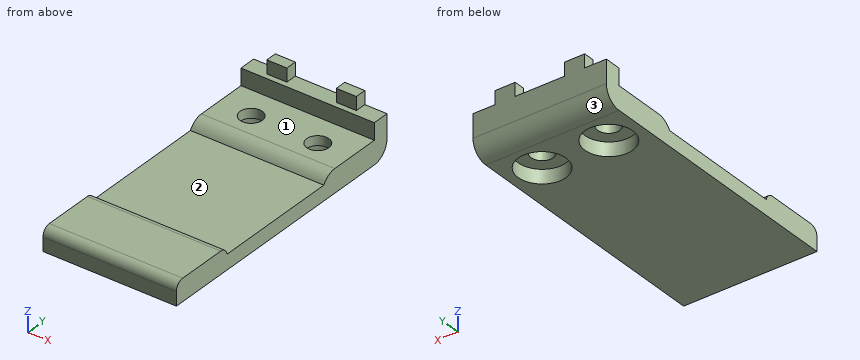
from build123d import *

# Parameters (mm, degrees)
F0_W        = 24
F0_H        = 12
F0_H_2      = 23
F0_R        = 4.3
F0_H_3      = 3
F1_DEPTH    = 2.7
F0_R_2      = 2
F2_DEPTH    = 4.2
F3_DEPTH    = 2.5
F4_DEPTH    = 7.2
F5_W        = 3.6
F5_H        = 2
F6_DEPTH    = 2.4
F7_T1_DEPTH = 39
F7_T3_DEPTH = 36.9903810568
F8_DEPTH    = 4
F9_T1_DEPTH = 31.4330343737
F9_T3_DEPTH = 31.5


# Not quite as in the source:
# - a fillet or chamfer that OpenCascade refuses, or shapes differently, is made with other operations: its cross-section is extruded or revolved along the edge and cut away or added


with BuildPart() as f1:
    # F0 (on Top) → F1 (new body)
    with BuildSketch(Plane.XY):
        with Locations((12, -44)):
            Rectangle(F0_W, F0_H)
        with Locations((12, -26.5)):
            Rectangle(F0_W, F0_H_2)
        with Locations((12, -9)):
            Rectangle(F0_W, F0_H)
        with Locations((6, -8.5)):
            Circle(F0_R, mode=Mode.SUBTRACT)
        with Locations((18, -8.5)):
            Circle(F0_R, mode=Mode.SUBTRACT)
        with Locations((12, -1.5)):
            Rectangle(F0_W, F0_H_3)
    extrude(amount=F1_DEPTH)

    # F0 (on Top) → F2 (join)
    with BuildSketch(Plane.XY):
        with Locations((12, -1.5)):
            Rectangle(F0_W, F0_H_3)
        with Locations((12, -9)):
            Rectangle(F0_W, F0_H)
        with Locations((6, -8.5)):
            Circle(F0_R, mode=Mode.SUBTRACT)
        with Locations((18, -8.5)):
            Circle(F0_R, mode=Mode.SUBTRACT)
        with Locations((6, -8.5)):
            Circle(F0_R)
        with Locations((6, -8.5)):
            Circle(F0_R_2, mode=Mode.SUBTRACT)
        with Locations((18, -8.5)):
            Circle(F0_R)
        with Locations((18, -8.5)):
            Circle(F0_R_2, mode=Mode.SUBTRACT)
    extrude(amount=F2_DEPTH)

    # F0 (on Top) → F3 (cut)
    with BuildSketch(Plane.XY):
        with Locations((6, -8.5)):
            Circle(F0_R)
        with Locations((6, -8.5)):
            Circle(F0_R_2, mode=Mode.SUBTRACT)
        with Locations((18, -8.5)):
            Circle(F0_R)
        with Locations((18, -8.5)):
            Circle(F0_R_2, mode=Mode.SUBTRACT)
    extrude(amount=F3_DEPTH, mode=Mode.SUBTRACT)

    # F0 (on Top) → F4 (join)
    with BuildSketch(Plane.XY):
        with Locations((12, -1.5)):
            Rectangle(F0_W, F0_H_3)
    extrude(amount=F4_DEPTH)

    # F5 (on face) → F6 (join)
    with BuildSketch(Plane.XY.offset(7.2)):
        with Locations((5.7, -1)):
            Rectangle(F5_W, F5_H)
        with Locations((18.2, -1)):
            Rectangle(F5_W, F5_H)
    extrude(amount=F6_DEPTH)

    # F7: fillet of radius 3 on 2 edges, made by hand

    # F7_s2 → F7_t1 (cut)
    with BuildSketch(Plane.YZ.offset(-7.5)):
        with BuildLine():
            ThreePointArc((-3, 0), (-0.8786796564, 0.8786796564), (0, 3))
            Line((0, 3), (0, 0))
            Line((0, 0), (-3, 0))
        make_face()
    extrude(amount=F7_T1_DEPTH, mode=Mode.SUBTRACT)

    # F7_s4 → F7_t3 (cut)
    with BuildSketch(Plane.YZ.offset(-6.4951905284)):
        with BuildLine():
            ThreePointArc((-12.4019237886, 4.2), (-13.9019237886, 3.7980762114), (-15, 2.7))
            Line((-15, 2.7), (-15, 4.2))
            Line((-15, 4.2), (-12.4019237886, 4.2))
        make_face()
    extrude(amount=F7_T3_DEPTH, mode=Mode.SUBTRACT)

    # F0 (on Top) → F8 (join)
    with BuildSketch(Plane.XY):
        with Locations((12, -44)):
            Rectangle(F0_W, F0_H)
    extrude(amount=F8_DEPTH)

    # F9: fillet of radius 1.5 on 2 edges, made by hand

    # F9_s2 → F9_t1 (cut)
    with BuildSketch(Plane.YZ.offset(-3.7165171868)):
        with BuildLine():
            ThreePointArc((-38, 2.7), (-38.4991859918, 3.6291589791), (-39.4866068747, 4))
            Line((-39.4866068747, 4), (-38, 4))
            Line((-38, 4), (-38, 2.7))
        make_face()
    extrude(amount=F9_T1_DEPTH, mode=Mode.SUBTRACT)

    # F9_s4 → F9_t3 (cut)
    with BuildSketch(Plane.YZ.offset(-3.75)):
        with BuildLine():
            ThreePointArc((-50, 2.5), (-49.5606601718, 3.5606601718), (-48.5, 4))
            Line((-48.5, 4), (-50, 4))
            Line((-50, 4), (-50, 2.5))
        make_face()
    extrude(amount=F9_T3_DEPTH, mode=Mode.SUBTRACT)


solid = f1.part
Can you work these out from the model? Positions are in its coordinate system, mm. Face numbers are marked on the shaded views. A direction names the side the tool comes from. Coordinates: 2 decimals unless noted, no trailing zeros. Loops run counter-clockwise (first coordinate to the right, second up) from the corner with the lowest first, then second, coordinate; pieces in that order, holes last. Notation, with made-up numbers: (-30, 62.25) - (-18, 62.25) arc R31 ccw to (-18, 87.25) - close; hole circle Ø10 at (80, 69.5). An arc over 180 degrees is marked (long way). Put each result on its own line as item: value. Start each with the question number.
Item 1: Suppose I cut it at A-A (y = -8.5). Please give me the cut outline in (x, z), and give its area (3 significant figures).
Item 2: Which directions (+Z, -Z, +X, -X, +Y, -Y) give clear straight access to the entire face, cutting with the end or side of a thin tool? Please do the marked faces 1, 2 and 3.
Item 3: For pin 1 (2.5 mm diameter, centred on x = 19, y = -8, fed in from -Z); pin 2 (4.5 mm diameter, centred on x = 18, y = -9, fed in from +Z); pin 3 (1.9 mm diameter, centred on x = 6.5, z = 9, fed in from -Y), each with a flat end and sliding along its axis, tell me the tip position at first contact or that it passes through.
Item 4: Suppose I cut it at B-B (z = 8.5). Please give me the cut outline in (x, y), and give its area (3 significant figures).
Item 5: Suppose I cut it at C-C (x = 18). Please give me the cut outline in (y, z), and give its area (3 significant figures).
Item 6: If I drill on line 1 along Z through (x, y) = (15.5, -19); line 2 along Z through (x, y) = (22.25, -6.5); line 3 along Y through (x, z) = (18, 1.2), over which ranges is the centre line in solid material (lowest first)?
Item 7: Suppose I cut it at D-D (x = 15.25). Please give me the cut outline in (y, z), and give its area (3 significant figures).
Here are the results:
1. outline: (0, 0) - (1.7, 0) - (1.7, 2.5) - (4, 2.5) - (4, 4.2) - (0, 4.2) - close; (8, 2.5) - (10.3, 2.5) - (10.3, 0) - (13.7, 0) - (13.7, 2.5) - (16, 2.5) - (16, 4.2) - (8, 4.2) - close; (20, 2.5) - (22.3, 2.5) - (22.3, 0) - (24, 0) - (24, 4.2) - (20, 4.2) - close
1. area: 44.2 mm²
2. face 1: +Z, +X, -X, -Y
2. face 2: +Z, +X, -X
2. face 3: -Z, +X, -X, +Y
3. pin 1: z = 2.5
3. pin 2: z = 4.2
3. pin 3: y = -2
4. outline: (3.9, -2) - (7.5, -2) - (7.5, 0) - (3.9, 0) - close; (16.4, -2) - (20, -2) - (20, 0) - (16.4, 0) - close
4. area: 14.4 mm²
5. outline: (-50, 0) - (-12.8, 0) - (-12.8, 2.5) - (-10.5, 2.5) - (-10.5, 4.2) - (-12.4, 4.2) arc R3 ccw to (-15, 2.7) - (-38, 2.7) arc R1.5 ccw to (-39.49, 4) - (-48.5, 4) arc R1.5 ccw to (-50, 2.5) - close; (-6.5, 2.5) - (-4.2, 2.5) - (-4.2, 0) - (-3, 0) arc R3 ccw to (0, 3) - (0, 9.6) - (-2, 9.6) - (-2, 7.2) - (-3, 7.2) - (-3, 4.2) - (-6.5, 4.2) - close
5. area: 155 mm²
6. line 1: 0 to 2.7
6. line 2: 0 to 4.2
6. line 3: -50 to -12.8, -4.2 to -0.6
7. outline: (-50, 0) - (-11.81, 0) - (-11.81, 2.5) - (-5.19, 2.5) - (-5.19, 0) - (-3, 0) arc R3 ccw to (0, 3) - (0, 7.2) - (-3, 7.2) - (-3, 4.2) - (-12.4, 4.2) arc R3 ccw to (-15, 2.7) - (-38, 2.7) arc R1.5 ccw to (-39.49, 4) - (-48.5, 4) arc R1.5 ccw to (-50, 2.5) - close
7. area: 162 mm²
